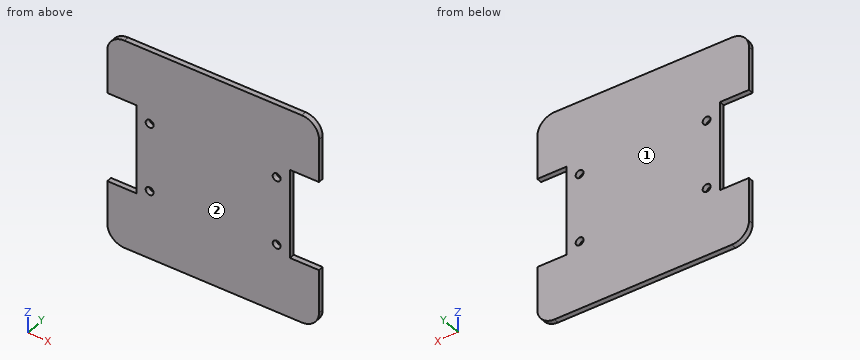
```python
from build123d import *

# Parameters (mm, degrees)
SKETCH1_R           = 1.5
BOSS_EXTRUDE1_DEPTH = 2


with BuildPart() as part:
    # Sketch1 → Boss-Extrude1 (new body)
    with BuildSketch(Plane(origin=(0, 0, 0), x_dir=(1, 0, 0), z_dir=(0, 1, 0))):
        with BuildLine():
            Line((6.5, 0), (73.5, 0))
            ThreePointArc((73.5, 0), (78.096194078, 1.903805922), (80, 6.5))
            Line((80, 6.5), (80, 23))
            Line((80, 23), (69, 23))
            Line((69, 23), (69, 57))
            Line((69, 57), (80, 57))
            Line((80, 57), (80, 73.5))
            ThreePointArc((80, 73.5), (78.096194078, 78.096194078), (73.5, 80))
            Line((73.5, 80), (6.5, 80))
            ThreePointArc((6.5, 80), (1.903805922, 78.096194078), (0, 73.5))
            Line((0, 73.5), (0, 57))
            Line((0, 57), (11, 57))
            Line((11, 57), (11, 23))
            Line((11, 23), (0, 23))
            Line((0, 23), (0, 6.5))
            ThreePointArc((0, 6.5), (1.903805922, 1.903805922), (6.5, 0))
        make_face()
        with Locations(Location((16, 54, 0), (0, 0, 270))):
            Circle(SKETCH1_R, mode=Mode.SUBTRACT)
        with Locations(Location((16, 28, 0), (0, 0, 270))):
            Circle(SKETCH1_R, mode=Mode.SUBTRACT)
        with Locations(Location((64, 28, 0), (0, 0, 90))):
            Circle(SKETCH1_R, mode=Mode.SUBTRACT)
        with Locations(Location((64, 54, 0), (0, 0, 90))):
            Circle(SKETCH1_R, mode=Mode.SUBTRACT)
    extrude(amount=BOSS_EXTRUDE1_DEPTH)


solid = part.part
```
Can you work these out from the model? Positions are in its coordinate system, mm. Face numbers are marked on the shaded views. Round coordinates to 2 decimals unless told otherwise and drop trailing zeros. Loops run counter-clockwise (first coordinate to the right, second up) from the corner with the lowest first, then second, coordinate; pieces in that order, holes last. Notation, with made-up numbers: M 24.25,22 L 71.25,22 A28 ccw 71.25,55 Z; hole C 1.25,41 d11. An arc over 180 degrees is marked long. Write item = value, one per line. Start each with the question number.
(1) I'm going to push flat-ended pins straight in: P1, Ø2.5, axis at x = 64, z = -54, coming from the -Y side; P2, Ø0.6, axis at y = 1, z = -43.5, coming from the +X side; P3, Ø1, axis at x = 5, y = 1, coming from the -Z side; P4, Ø0.6, axis at x = 74.5, y = 1, coming from the +Z side. Where does each tip first touch, or does it pass through?
(2) Suppose I cut it at C-C on y = 1.05. Write out the boundary of the cut face in (x, z), plus the area to 3 significant figures.
(3) Suppose I cut it at A-A on x = 16. Write out the boundary of the cut face in (y, z), plus the area to 3 significant figures.
(4) Suppose I cut it at D-D on x = 8. Write out the boundary of the cut face in (y, z).
(5) Suppose I cut it at B-B on z = -28. Write out the boundary of the cut face in (x, y), plus the area to 3 significant figures.
(6) I need wall thicknesses on line 1 along X through (y, z) = (1.25, -28); line 2 along Z through (x, y) = (64, 1.2); line 3 along Z through (x, y) = (71, 1.25). Which ranges of each line are inside material? Lowest first, please.
(7) If we mould it in two halves opening along Y, with no side actions, what happens to the marked faces 1 and 2? For each: released by +Y, released by -Y, zero draft, split by the parting line, or undercut.
Answer block:
q1.P1 = through
q1.P2 = 69
q1.P3 = -79.92
q1.P4 = -0.04
q2.outline = M 0,-73.5 A6.5 ccw 6.5,-80 L 73.5,-80 A6.5 ccw 80,-73.5 L 80,-57 L 69,-57 L 69,-23 L 80,-23 L 80,-6.5 A6.5 ccw 73.5,0 L 6.5,0 A6.5 ccw 0,-6.5 L 0,-23 L 11,-23 L 11,-57 L 0,-57 Z; hole C 16,-54 d3; hole C 16,-28 d3; hole C 64,-54 d3; hole C 64,-28 d3
q2.area = 5,590 mm²
q3.outline = M 0,-80 L 2,-80 L 2,-55.5 L 0,-55.5 Z; M 0,-52.5 L 2,-52.5 L 2,-29.5 L 0,-29.5 Z; M 0,-26.5 L 2,-26.5 L 2,0 L 0,0 Z
q3.area = 148 mm²
q4.outline = M 0,-80 L 2,-80 L 2,-57 L 0,-57 Z; M 0,-23 L 2,-23 L 2,0 L 0,0 Z
q5.outline = M 11,0 L 14.5,0 L 14.5,2 L 11,2 Z; M 17.5,0 L 62.5,0 L 62.5,2 L 17.5,2 Z; M 65.5,0 L 69,0 L 69,2 L 65.5,2 Z
q5.area = 104 mm²
q6.line_1 = 11 to 14.5, 17.5 to 62.5, 65.5 to 69
q6.line_2 = -80 to -55.5, -52.5 to -29.5, -26.5 to 0
q6.line_3 = -80 to -57, -23 to 0
q7.face_1 = released by +Y
q7.face_2 = released by -Y
